Part model, mm, in its own coordinate system. A direction names the side the tool comes from. Round coordinates to 2 decimals unless told otherwise and drop trailing zeros. Write each loop counter-clockwise with the first axis right and the second up, starting at its lowest first coordinate (ties: lowest second). Pieces come first, ordered by that corner, then holes.
1) Drill centre lines: L1, parallel to Y at x = 14, z = 0.65; L2, parallel to X at y = -3.5, z = 7.5; L3, parallel to Y at x = 56, z = 0.7. Where is each one in solid material? Low to high.
2) Which spindle directions (+Z, -Z, +X, -X, +Y, -Y) get a long thin tool onto all of the face, cutting with end or side? Do faces 4 (the flat face through (3, -10, 5)), 5 (the flat face through (30, 0, 4)), 6 (the flat face through (27, -2, 8)), 7 (the flat face through (57, -50, 5)), 8 (the flat face through (54, -46, 3)). Say none if no direction does.
3) Flat gauge pins, fed straight in: pin 1 (2 mm diameter, centred on x = 12, y = -42.5, fed in from -Z); pin 2 (1.5 mm diameter, centred on y = -42.5, z = 7.5, fed in from -X); pin 3 (10 mm diameter, centred on x = 25, y = -30, fed in from +Z); pin 4 (4 mm diameter, centred on x = 48, y = -17.5, fed in from +Z). Where does each tip first touch, or does it go through?
4) Pull direction X, two halves, no side cores. Call faces 1 (the flat face through (50, -3, 5)), 2 (the cylindrical face through (12.16, -41.26, 1.48)), 3 (the flat face through (39, -54, 10)): +X half, -X half, draft (parallel to the pull), parting line (faces both ways), or undercut.
5) Saw through at A-A on y = -30. Write the cut outline in (x, z).
6) Saw through at B-B on x = 20. Write the cut outline in (y, z).
```python
from build123d import *

# Parameters (mm, degrees)
SKETCH_1_W             = 60
SKETCH_1_H             = 60
EXTRUDE_1_DEPTH        = 10
SKETCH_2_R             = 25.25
CUT_EXTRUDE_1_DEPTH    = 8
SKETCH_4_W             = 10
SKETCH_4_H             = 10
CUT_EXTRUDE_3_DEPTH    = 11
FILLET_1_R             = 6
FILLET_2_R             = 2
SKETCH_5_R             = 1.75
CUT_EXTRUDE_4_DEPTH    = 11
EXTRUDE_2_DEPTH        = 1
FILLET_5_R             = 2
HOLE_WIZARD_M3_2_D     = 2.5
HOLE_WIZARD_M3_2_DEPTH = 7.5
HOLE_WIZARD_M3_2_TIP   = 0.751075774
SKETCH_21_R            = 1.25
SKETCH_21_W            = 5
SKETCH_21_H            = 5
SKETCH_21_W_2          = 6
SKETCH_21_H_2          = 6
CUT_EXTRUDE_9_DEPTH    = 10
SKETCH_23_R            = 1.25
SKETCH_23_W            = 5
SKETCH_23_H            = 12
CUT_EXTRUDE_10_DEPTH   = 10
SKETCH_25_R            = 2.75
CUT_EXTRUDE_11_DEPTH   = 3
FILLET_6_R             = 2


with BuildPart() as part:
    # 草图1 → 凸台-拉伸1 (new body)
    with BuildSketch(Plane.XY):
        with Locations((30, -30)):
            Rectangle(SKETCH_1_W, SKETCH_1_H)
    extrude(amount=EXTRUDE_1_DEPTH)

    # 草图2 → 切除-拉伸1 (cut)
    with BuildSketch(Plane.XY.offset(10)):
        with Locations((30, -30)):
            Circle(SKETCH_2_R)
    extrude(amount=-CUT_EXTRUDE_1_DEPTH, mode=Mode.SUBTRACT)

    # 草图4 → 切除-拉伸3 (cut, through all)
    with BuildSketch(Plane(origin=(0, 0, 0), x_dir=(-1, 0, 0), z_dir=(0, 0, -1))):
        with Locations((-5, -5)):
            Rectangle(SKETCH_4_W, SKETCH_4_H)
        with Locations((-55, -5)):
            Rectangle(SKETCH_4_W, SKETCH_4_H)
        with Locations((-5, -55)):
            Rectangle(SKETCH_4_W, SKETCH_4_H)
        with Locations((-55, -55)):
            Rectangle(SKETCH_4_W, SKETCH_4_H)
    extrude(amount=-CUT_EXTRUDE_3_DEPTH, mode=Mode.SUBTRACT)

    # 圆角1
    fillet_1_edges = [part.edges().sort_by_distance(p)[0] for p in [
        (50, -50, 5),
        (10, -50, 5),
        (10, -10, 5),
        (50, -10, 5),
    ]]
    fillet(fillet_1_edges, radius=FILLET_1_R)

    # 圆角2
    fillet_2_edges = [part.edges().sort_by_distance(p)[0] for p in [
        (60, -50, 5),
        (50, -60, 5),
        (0, -50, 5),
        (10, -60, 5),
        (10, 0, 5),
        (0, -10, 5),
        (60, -10, 5),
        (50, 0, 5),
    ]]
    fillet(fillet_2_edges, radius=FILLET_2_R)

    # 草图5 → 切除-拉伸4 (cut, through all)
    with BuildSketch(Plane(origin=(0, 0, 0), x_dir=(-1, 0, 0), z_dir=(0, 0, -1))):
        with Locations((-4, -14)):
            Circle(SKETCH_5_R)
        with Locations((-14, -56)):
            Circle(SKETCH_5_R)
        with Locations((-56, -46)):
            Circle(SKETCH_5_R)
        with Locations((-46, -4)):
            Circle(SKETCH_5_R)
    extrude(amount=-CUT_EXTRUDE_4_DEPTH, mode=Mode.SUBTRACT)

    # 草图15 → 凸台-拉伸2 (add)
    with BuildSketch(Plane.XY.offset(2)):
        with BuildLine():
            Line((46.393030976, -15.584888892), (49.013896395, -13.385721686))
            ThreePointArc((49.013896395, -13.385721686), (50.732040439, -15.58663817), (52.196675107, -17.963799843))
            Line((52.196675107, -17.963799843), (49.25, -19.665063509))
            ThreePointArc((49.25, -19.665063509), (45.952119889, -18.933941091), (46.393030976, -15.584888892))
        make_face()
        with BuildLine():
            Line((13.606969024, -15.584888892), (10.986103605, -13.385721686))
            ThreePointArc((10.986103605, -13.385721686), (9.267959561, -15.58663817), (7.803324893, -17.963799843))
            Line((7.803324893, -17.963799843), (10.75, -19.665063509))
            ThreePointArc((10.75, -19.665063509), (14.047880111, -18.933941091), (13.606969024, -15.584888892))
        make_face()
        with BuildLine():
            Line((46.393030976, -44.415111108), (49.013896395, -46.614278314))
            ThreePointArc((49.013896395, -46.614278314), (50.732040439, -44.41336183), (52.196675107, -42.036200157))
            Line((52.196675107, -42.036200157), (49.25, -40.334936491))
            ThreePointArc((49.25, -40.334936491), (45.952119889, -41.066058909), (46.393030976, -44.415111108))
        make_face()
        with BuildLine():
            Line((10.75, -40.334936491), (7.803324893, -42.036200157))
            ThreePointArc((7.803324893, -42.036200157), (9.267959561, -44.41336183), (10.986103605, -46.614278314))
            Line((10.986103605, -46.614278314), (13.606969024, -44.415111108))
            ThreePointArc((13.606969024, -44.415111108), (14.047880111, -41.066058909), (10.75, -40.334936491))
        make_face()
    extrude(amount=EXTRUDE_2_DEPTH)

    # 圆角5
    fillet_5_edges = [part.edges().sort_by_distance(p)[0] for p in [
        (10.986103605, -13.385721686, 2.5),
        (7.803324893, -17.963799843, 2.5),
        (52.196675107, -17.963799843, 2.5),
        (49.013896395, -13.385721686, 2.5),
        (49.013896395, -46.614278314, 2.5),
        (52.196675107, -42.036200157, 2.5),
        (7.803324893, -42.036200157, 2.5),
        (10.986103605, -46.614278314, 2.5),
    ]]
    fillet(fillet_5_edges, radius=FILLET_5_R)

    # M3 螺纹孔2
    with Locations(Plane.XY.offset(3)):
        with Locations((12, -17.5), (12, -42.5), (48, -17.5), (48, -42.5)):
            Hole(HOLE_WIZARD_M3_2_D / 2, depth=HOLE_WIZARD_M3_2_DEPTH)
            with Locations((0, 0, -(HOLE_WIZARD_M3_2_DEPTH + HOLE_WIZARD_M3_2_TIP / 2))):  # 118° drill point
                Cone(0, HOLE_WIZARD_M3_2_D / 2, HOLE_WIZARD_M3_2_TIP, mode=Mode.SUBTRACT)

    # 草图21 → 切除-拉伸9 (cut)
    with BuildSketch(Plane(origin=(0, 0, 0), x_dir=(1, 0, 0), z_dir=(0, 1, 0))):
        with Locations((17.5, -7.5)):
            Circle(SKETCH_21_R)
        with Locations((42.5, -7.5)):
            Circle(SKETCH_21_R)
        with Locations((36.5, -7.5)):
            Rectangle(SKETCH_21_W, SKETCH_21_H)
        with Locations((24, -7)):
            Rectangle(SKETCH_21_W_2, SKETCH_21_H_2)
    extrude(amount=-CUT_EXTRUDE_9_DEPTH, mode=Mode.SUBTRACT)

    # 草图23 → 切除-拉伸10 (cut)
    with BuildSketch(Plane.ZY):
        with Locations((7.5, -17.5)):
            Circle(SKETCH_23_R)
        with Locations((7.5, -42.5)):
            Circle(SKETCH_23_R)
        with Locations((7.5, -30)):
            Rectangle(SKETCH_23_W, SKETCH_23_H)
    extrude(amount=-CUT_EXTRUDE_10_DEPTH, mode=Mode.SUBTRACT)

    # 草图25 → 切除-拉伸11 (cut)
    with BuildSketch(Plane(origin=(0, 0, 0), x_dir=(-1, 0, 0), z_dir=(0, 0, -1))):
        with Locations((-4, -14)):
            Circle(SKETCH_25_R)
        with Locations((-46, -4)):
            Circle(SKETCH_25_R)
        with Locations((-56, -46)):
            Circle(SKETCH_25_R)
        with Locations((-14, -56)):
            Circle(SKETCH_25_R)
    extrude(amount=-CUT_EXTRUDE_11_DEPTH, mode=Mode.SUBTRACT)

    # 圆角6
    fillet_6_edges = [part.edges().sort_by_distance(p)[0] for p in [
        (21, -3.204211557, 4),
        (27, -2.464425621, 4),
        (34, -2.534422396, 5),
        (39, -3.204211557, 5),
        (2.736614456, -36, 5),
        (2.736614456, -24, 5),
    ]]
    fillet(fillet_6_edges, radius=FILLET_6_R)


solid = part.part
```
Completed:
1. L1: y = -60 to -58.75, -53.25 to 0
1. L2: x = 10 to 16.25, 18.75 to 21, 27 to 34, 39 to 41.25, 43.75 to 44.32, 47.68 to 50
1. L3: y = -50 to -48.75, -43.25 to -10
2. face 4: +Z, -Z, -X, +Y
2. face 5: +Z, -Z, +X, -X, +Y
2. face 6: +Z, +Y
2. face 7: +Z, -Z, +X, -Y
2. face 8: -Z
3. pin 1: passes through
3. pin 2: stops at x = 51.49
3. pin 3: stops at z = 2
3. pin 4: stops at z = 3
4. face 1: +X half
4. face 2: undercut
4. face 3: draft
5. outline: (0, 0) - (60, 0) - (60, 10) - (55.25, 10) - (55.25, 2) - (4.75, 2) - (4.75, 5) - (0, 5) - close
6. outline: (-60, 0) - (0, 0) - (0, 10) - (-6.81, 10) - (-6.81, 2) - (-53.19, 2) - (-53.19, 10) - (-60, 10) - close
